Source: CAD feature listing. Evaluate the final solid. Frame: model axes, mm. A direction names the side the tool comes from. Coordinates: 2 decimals unless noted, no trailing zeros. Order: outer loops, then holes, each group sorted by start corner. A loop starts at its lowest first (then second) coordinate and runs counter-clockwise, first axis right, second up. Notation, with made-up numbers: (13, -39.75) - (60, -39.75) arc R17 cw to (60, -7.75) - close; hole circle Ø7 at (-35, 87.5). An arc over 180 degrees is marked (long way). One line per question, with ' | ' between items. Start each with the question number.
(1) Line query: line 1 along Y through (x, z) = (0, 4.5); line 2 along X through (y, z) = (0.5, 27); line 3 along Y through (x, z) = (-14, 6.5). Output: solid intervals per line, ascending.
(2) Draft query along X for faces 5 (the flat face through (-6, -28, 5)), 6 (the flat face through (0, -23, 24)), 7 (the cylindrical face through (-0.234, 30.785, 5.07)). Return one class per face: +X half, -X half, draft (parallel to the pull), parting line (faces both ways), or undercut.
(3) Section A-A (x = 0). Return the cut outline in (y, z), then the cut area to 3 significant figures.
(4) Section C-C (y = 29). Return the cut outline in (x, z).
(5) Access query for faces 1 (the flat face through (-1.4, -27.6, 10)), 2 (the flat face through (6, -28, 5)), 3 (the flat face through (13.4, 17.64, 45.04)), 4 (the flat face through (-23, 0, 29)). Directions: +Z, -Z, +X, -X, +Y, -Y. A direction counts if a zero-diameter tool reaches every point of the face in a straight line with its end or side. Return the directions, or none.
(6) Section B-B (z = 27.5). Return the cut outline in (x, y), then the cut area to 3 significant figures.
(7) Contact query for flat-ended pins moving along their axis: P1, Ø3, axis at x = -16.5, z = 24, coming from the -Y side; P2, Ø5, axis at y = -28, z = 5, coming from the -X side; P3, Ø3, axis at x = 2.5, z = 24, coming from the +Y side. Output: stop coordinate, or through.
(8) Section D-D (x = -8.5). Return the cut outline in (y, z), then the cut area to 4 significant figures.
from build123d import *

# Parameters (mm, degrees)
MAIN_DEPTH           = 48
SKETCH2_R            = 16.7
MOTOR_HOLE_DEPTH     = 49
PULLEY_OUT_REACH     = 48
SKETCH3_W            = 10
SKETCH3_H            = 30
NUTS_DEPTH           = 6
M3_CLEARANCE_HOLE1_D = 3.6
BOSS_EXTRUDE2_DEPTH  = 10
M3_CLEARANCE_HOLE2_D = 3.6


with BuildPart() as part:
    # Sketch1 → Main (new body)
    with BuildSketch(Plane.XY):
        with BuildLine():
            Line((-15.5, 23), (15.5, 23))
            ThreePointArc((15.5, 23), (20.803300859, 20.803300859), (23, 15.5))
            Line((23, 15.5), (23, -15.5))
            ThreePointArc((23, -15.5), (20.803300859, -20.803300859), (15.5, -23))
            Line((15.5, -23), (-15.5, -23))
            ThreePointArc((-15.5, -23), (-20.803300859, -20.803300859), (-23, -15.5))
            Line((-23, -15.5), (-23, 15.5))
            ThreePointArc((-23, 15.5), (-20.803300859, 20.803300859), (-15.5, 23))
        make_face()
    extrude(amount=MAIN_DEPTH)

    # Sketch2 → Motor Hole (cut, through all)
    with BuildSketch(Plane(origin=(0, 0, 0), x_dir=(-1, 0, 0), z_dir=(0, 0, -1))):
        Circle(SKETCH2_R)
    extrude(amount=-MOTOR_HOLE_DEPTH, mode=Mode.SUBTRACT)

    # Sketch3 → Pulley Out (cut, up to next)
    with BuildSketch(Plane.ZY.offset(23), mode=Mode.PRIVATE) as pulley_out_sk1:
        with Locations((12, 0)):
            Rectangle(SKETCH3_W, SKETCH3_H)
    pulley_out_tool1 = extrude(pulley_out_sk1.sketch, amount=-PULLEY_OUT_REACH, mode=Mode.PRIVATE) & part.part
    add(pulley_out_tool1.solids().sort_by_distance((-23, 0, 12))[0], mode=Mode.SUBTRACT)

    # Sketch9 → Nuts (cut)
    with BuildSketch(Plane.XY.offset(48)):
        Polygon((-18.681980515, -14.439339828), (-16.63137085, -12.388730163), (-12.388730163, -16.63137085), (-14.439339828, -18.681980515), align=None)
        Polygon((18.681980515, 14.439339828), (16.63137085, 12.388730163), (12.388730163, 16.63137085), (14.439339828, 18.681980515), align=None)
    extrude(amount=-NUTS_DEPTH, mode=Mode.SUBTRACT)

    # M3 Clearance Hole1 (through all)
    with Locations(Plane(origin=(-20.803300859, -20.803300859, 45), x_dir=(-0.707106781, 0.707106781, 0), z_dir=(-0.707106781, -0.707106781, 0))):
        with Locations((0, 0)):
            Hole(M3_CLEARANCE_HOLE1_D / 2)

    # Sketch15 → Boss-Extrude2 (add)
    with BuildSketch(Plane(origin=(0, 0, 0), x_dir=(-1, 0, 0), z_dir=(0, 0, -1))):
        with BuildLine():
            Line((-6, -23), (6, -23))
            Line((6, -23), (6, -33))
            ThreePointArc((6, -33), (5.414213562, -34.414213562), (4, -35))
            Line((4, -35), (-4, -35))
            ThreePointArc((-4, -35), (-5.414213562, -34.414213562), (-6, -33))
            Line((-6, -33), (-6, -23))
        make_face()
        with BuildLine():
            Line((-4, 35), (4, 35))
            ThreePointArc((4, 35), (5.414213562, 34.414213562), (6, 33))
            Line((6, 33), (6, 23))
            Line((6, 23), (-6, 23))
            Line((-6, 23), (-6, 33))
            ThreePointArc((-6, 33), (-5.414213562, 34.414213562), (-4, 35))
        make_face()
    extrude(amount=-BOSS_EXTRUDE2_DEPTH)

    # M3 Clearance Hole2 (through all)
    with Locations(Plane(origin=(0, 0, 0), x_dir=(-1, 0, 0), z_dir=(0, 0, -1))):
        with Locations((0, -29), (0, 29)):
            Hole(M3_CLEARANCE_HOLE2_D / 2)


solid = part.part
Response values:
1) line 1: y = -35 to -30.8, -27.2 to -16.7, 16.7 to 27.2, 30.8 to 35 | line 2: x = -23 to -16.69, 16.69 to 23 | line 3: y = -23 to -9.1, 9.1 to 23
2) face 5: -X half | face 6: draft | face 7: undercut
3) outline: (-35, 0) - (-30.8, 0) - (-30.8, 10) - (-35, 10) - close; (-27.2, 0) - (-16.7, 0) - (-16.7, 48) - (-23, 48) - (-23, 10) - (-27.2, 10) - close; (16.7, 0) - (27.2, 0) - (27.2, 10) - (23, 10) - (23, 48) - (16.7, 48) - close; (30.8, 0) - (35, 0) - (35, 10) - (30.8, 10) - close | area: 773 mm²
4) outline: (-6, 0) - (-1.8, 0) - (-1.8, 10) - (-6, 10) - close; (1.8, 0) - (6, 0) - (6, 10) - (1.8, 10) - close
5) face 1: +Z, +X, -X, -Y | face 2: +Z, -Z, +X, -Y | face 3: +Z | face 4: +Z, -Z, -X, +Y, -Y
6) outline: (-23, -15.5) arc R7.5 ccw to (-15.5, -23) - (15.5, -23) arc R7.5 ccw to (23, -15.5) - (23, 15.5) arc R7.5 ccw to (15.5, 23) - (-15.5, 23) arc R7.5 ccw to (-23, 15.5) - close; hole circle Ø33.4 at (0, 0) | area: 1,190 mm²
7) P1: stops at y = -23 | P2: stops at x = -6 | P3: stops at y = 23
8) outline: (-23, 0) - (-14.37, 0) - (-14.37, 7) - (-15, 7) - (-15, 17) - (-14.37, 17) - (-14.37, 48) - (-23, 48) - close; (14.37, 0) - (23, 0) - (23, 48) - (14.37, 48) - (14.37, 17) - (15, 17) - (15, 7) - (14.37, 7) - close | area: 815.5 mm²
